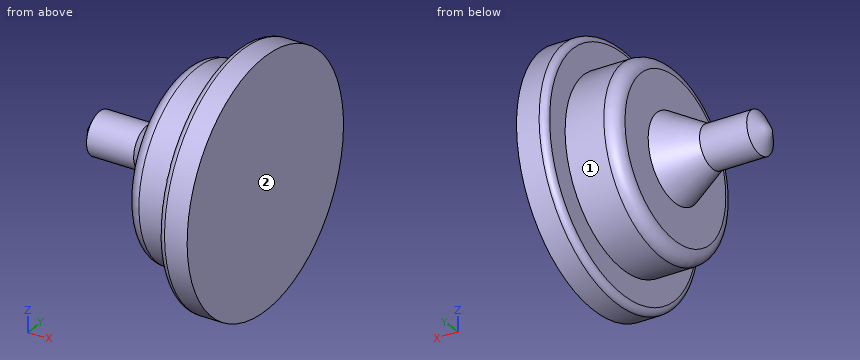
```python
from build123d import *


with BuildPart() as f1:
    # F0 (on Front) → F1 (revolve)
    with BuildSketch(Plane.XZ):
        with BuildLine():
            Line((27.5, 0), (27.5, 19))
            Line((27.5, 19), (24, 19))
            ThreePointArc((24, 19), (23.292893, 18.707107), (23, 18))
            Line((23, 18), (23, 14.25))
            Line((23, 14.25), (17, 14.25))
            ThreePointArc((17, 14.25), (15.585786, 13.664214), (15, 12.25))
            Line((15, 12.25), (15, 6.612264))
            Line((15, 6.612264), (9.176388, 3.25))
            Line((9.176388, 3.25), (1.876388, 3.25))
            Line((1.876388, 3.25), (0, 0))
            Line((0, 0), (27.5, 0))
        make_face()
    revolve(axis=Axis((13.75, 0, 0), (1, 0, 0)))


solid = f1.part
```
The listing builds one solid part. Answer for the finished solid, in the listing's coordinates (mm). Face numbers are marked on the shaded views. A direction names the side the tool comes from. Round coordinates to 2 decimals unless told otherwise and drop trailing zeros. Loops run counter-clockwise (first coordinate to the right, second up) from the corner with the lowest first, then second, coordinate; pieces in that order, holes last.
Q1. Find the intervals of material crossed by line 1 (X direction, y = 12, z = 10); line 2 (X direction, y = -7, z = 1); line 3 (Z direction, x = 18.25, y = 8), in increasing order.
Q2. Given pin 1 Ø2 at (x, y) = (20, 4.5) entering from -Z; pin 2 Ø6 at (x, z) = (19, -7.5) entering from -Y; pin 3 Ø6 at (x, z) = (13.5, -9.5) entering from +Y, each flat-ended and moving along its own axis, determine where each tip first touches the part or whether it passes through.
Q3. Which of the six approach directions +Z, -Z, +X, -X, +Y, -Y give full straight-line access (tool end or side, diameter ignored) to the marked faces 1 and 2?
Q4. Section A-A, the plane x = 21.5 is taken. Determine the outline of the cut face in (y, z), then the cut area to 3 significant figures.
Q5. Section B-B, the plane x = 5.5 is taken. Determine the outline of the cut face in (y, z).
Completed:
1. line 1: x = 23 to 27.5
1. line 2: x = 15 to 27.5
1. line 3: z = -11.79 to 11.79
2. pin 1: stops at z = -13.81
2. pin 2: stops at y = -13.52
2. pin 3: stops at y = 11.6
3. face 1: -X
3. face 2: +Z, -Z, +X, +Y, -Y
4. outline: circle Ø28.5 at (0, 0)
4. area: 638 mm2
5. outline: circle Ø6.5 at (0, 0)
